Source: CAD feature listing. Evaluate the final solid. Frame: model axes, mm. Coordinates: 2 decimals unless noted, no trailing zeros. Write each loop counter-clockwise with the first axis right and the second up, starting at its lowest first coordinate (ties: lowest second). Pieces come first, ordered by that corner, then holes. Notation, with made-up numbers: M 64,40 L 95,40 A5 cw 95,46 Z; hole C 54,85 d2. An arc over 180 degrees is marked long. Write item = value, one per line. Start each with the question number.
1. Pin query (flat end, axial travel): pin 1 Ø1.6 at (y, z) = (-1.5, -1) entering from -X; pin 2 Ø0.9 at (x, y) = (26.5, -2) entering from -Z; pin 3 Ø0.9 at (y, z) = (-1.5, -1.5) entering from +X. Return the tip coordinate at first contact, or that it passes through.
2. Section query A-A (y = -0.6). Output: boundary loops of the cut face in (x, z), then the cut area to 3 significant figures.
3. Line query: line 1 along Z through (x, y) = (201, -2). Output: solid intervals per line, ascending.
4. Section query B-B (x = 261). Output: boundary loops of the cut face in (y, z), then the cut area to 3 significant figures.
```python
from build123d import *

# Parameters (mm, degrees)
F0_W     = 20.32
F0_H     = 3.1
F1_DEPTH = 3.1


with BuildPart() as f1:
    # F0 (on Front) → F1 (new body)
    with BuildSketch(Plane.XZ):
        with BuildLine():
            Line((150.0847015591, 26.4639822764), (0, 0))
            Line((0, 0), (66.04, 0))
            Line((66.04, 0), (86.36, 0))
            Line((86.36, 0), (152.4, 0))
            ThreePointArc((152.4, 0), (151.8200719892, 13.2825351947), (150.0847015591, 26.4639822764))
        make_face()
        with BuildLine():
            Line((0, 152.4), (0, 0))
            Line((0, 0), (26.4639822764, 150.0847015591))
            ThreePointArc((26.4639822764, 150.0847015591), (13.2825351947, 151.8200719892), (0, 152.4))
        make_face()
        with BuildLine():
            Line((26.4639822764, 150.0847015591), (0, 0))
            Line((0, 0), (52.1238698428, 143.2091554078))
            ThreePointArc((52.1238698428, 143.2091554078), (39.4440224736, 147.2070959265), (26.4639822764, 150.0847015591))
        make_face()
        with BuildLine():
            Line((52.1238698428, 143.2091554078), (0, 0))
            Line((0, 0), (76.2, 131.9822715367))
            ThreePointArc((76.2, 131.9822715367), (64.4070230893, 138.1213067444), (52.1238698428, 143.2091554078))
        make_face()
        with BuildLine():
            Line((76.2, 131.9822715367), (0, 0))
            Line((0, 0), (97.9608317162, 116.7451731313))
            ThreePointArc((97.9608317162, 116.7451731313), (87.4130488999, 124.8387715496), (76.2, 131.9822715367))
        make_face()
        with BuildLine():
            Line((97.9608317162, 116.7451731313), (0, 0))
            Line((0, 0), (116.7451731313, 97.9608317162))
            ThreePointArc((116.7451731313, 97.9608317162), (107.7630734528, 107.7630734528), (97.9608317162, 116.7451731313))
        make_face()
        with BuildLine():
            Line((116.7451731313, 97.9608317162), (0, 0))
            Line((0, 0), (131.9822715367, 76.2))
            ThreePointArc((131.9822715367, 76.2), (124.8387715496, 87.4130488999), (116.7451731313, 97.9608317162))
        make_face()
        with BuildLine():
            Line((131.9822715367, 76.2), (0, 0))
            Line((0, 0), (143.2091554078, 52.1238698428))
            ThreePointArc((143.2091554078, 52.1238698428), (138.1213067444, 64.4070230893), (131.9822715367, 76.2))
        make_face()
        with BuildLine():
            Line((143.2091554078, 52.1238698428), (0, 0))
            Line((0, 0), (150.0847015591, 26.4639822764))
            ThreePointArc((150.0847015591, 26.4639822764), (147.2070959265, 39.4440224736), (143.2091554078, 52.1238698428))
        make_face()
        with Locations((76.2, -1.55)):
            Rectangle(F0_W, F0_H)
        with BuildLine():
            Line((304.8, 152.4), (0, 152.4))
            ThreePointArc((0, 152.4), (13.2825351947, 151.8200719892), (26.4639822764, 150.0847015591))
            ThreePointArc((26.4639822764, 150.0847015591), (39.4440224736, 147.2070959265), (52.1238698428, 143.2091554078))
            ThreePointArc((52.1238698428, 143.2091554078), (64.4070230893, 138.1213067444), (76.2, 131.9822715367))
            ThreePointArc((76.2, 131.9822715367), (87.4130488999, 124.8387715496), (97.9608317162, 116.7451731313))
            ThreePointArc((97.9608317162, 116.7451731313), (107.7630734528, 107.7630734528), (116.7451731313, 97.9608317162))
            ThreePointArc((116.7451731313, 97.9608317162), (124.8387715496, 87.4130488999), (131.9822715367, 76.2))
            ThreePointArc((131.9822715367, 76.2), (138.1213067444, 64.4070230893), (143.2091554078, 52.1238698428))
            ThreePointArc((143.2091554078, 52.1238698428), (147.2070959265, 39.4440224736), (150.0847015591, 26.4639822764))
            ThreePointArc((150.0847015591, 26.4639822764), (151.8200719892, 13.2825351947), (152.4, 0))
            Line((152.4, 0), (218.44, 0))
            Line((218.44, 0), (238.76, 0))
            Line((238.76, 0), (301.7, 0))
            Line((301.7, 0), (304.8, 0))
            Line((304.8, 0), (304.8, 25.4))
            Line((304.8, 25.4), (304.8, 152.4))
        make_face()
        with Locations((228.6, -1.55)):
            Rectangle(F0_W, F0_H)
    extrude(amount=F1_DEPTH)


solid = f1.part
```
Results are:
q1.pin_1 = 66.04
q1.pin_2 = 0
q1.pin_3 = 238.76
q2.outline = M 0,0 L 66.04,0 L 66.04,-3.1 L 86.36,-3.1 L 86.36,0 L 218.44,0 L 218.44,-3.1 L 238.76,-3.1 L 238.76,0 L 304.8,0 L 304.8,152.4 L 0,152.4 Z
q2.area = 46,600 mm^2
q3.line_1 = 0 to 152.4
q4.outline = M -3.1,0 L 0,0 L 0,152.4 L -3.1,152.4 Z
q4.area = 472 mm^2
